Verification items for the finished model (mm, model axes). Give positions to 0.01 mm unless a question says otherwise; leave off trailing zeros. Loops run counter-clockwise (first coordinate to the right, second up) from the corner with the lowest first, then second, coordinate; pieces in that order, holes last. Notation, with made-up numbers: (82, 52) - (106, 52) arc R15 ccw to (106, 72) - close; hole circle Ø2 at (6, -16.75). An arc over 180 degrees is marked (long way). One line per item, written item: value. Start each with the question number.
1. Sectioned sample at D-D (x = 1.95). Count the separate pieces of the cut face and the enclosed holes in it, plus the area to 3 significant figures.
2. Scan lines: L1, parallel to Z at x = 2.25, y = 41; L2, parallel to Y at x = 0.5, z = -64 (3 decimals); L3, parallel to Z at x = 1.9, y = 6.5 (3 decimals). Record each from-to range of solid material in increasing order. Write a range as [from, to].
3. Sectioned sample at C-C (z = -80.5). Record the cut outline in (x, y).
4. Gauge pin test, flat ends, axial feed: pin 1 (1.5 mm diameter, centred on x = 2, y = 7, fed in from +Z); pin 2 (1.5 mm diameter, centred on x = 2, y = 7, fed in from -Z); pin 3 (0.9 mm diameter, centred on x = 1, y = 6, fed in from +Z). Record the tip position at first contact, or that the pin passes through.
5. Sectioned sample at B-B (y = 6.5). Record the cut outline in (x, z) (3 decimals), plus the area to 3 significant figures.
6. Sectioned sample at A-A (z = -11). Record the cut outline in (x, y), plus the area to 3 significant figures.
Autodesk Inventor part; units mm, degrees
ref_plane "YZ Plane" through (0, 0, 0) normal (1, 0, 0) x (0, 1, 0)
ref_plane "XZ Plane" through (0, 0, 0) normal (0, 1, 0) x (-1, 0, 0)
ref_plane "XY Plane" through (0, 0, 0) normal (0, 0, 1) x (1, 0, 0)
sketch "Sketch1" plane through (0, 0, 0) normal (1, 0, 0) x (0, 1, 0)
  line L0 (18.4717, 7.7423) -> (30.7168, -6.8509)
  line L1 (75.6155, -60.3591) -> (73.4706, -62.1589)
  line L2 (73.4706, -62.1589) -> (61.2255, -47.5657) construction
  line L3 (16.3268, 5.9425) -> (18.4717, 7.7423)
  line L4 (30.7168, -6.8509) -> (28.5719, -8.6507)
  line L5 (63.3704, -45.7659) -> (61.2255, -47.5657)
  line L6 (30.7168, -6.8509) -> (63.3704, -45.7659) construction
  line L7 (63.3704, -45.7659) -> (75.6155, -60.3591)
  line L8 (61.2255, -47.5657) -> (45.895, -29.2956)
  line L9 (28.5719, -8.6507) -> (16.3268, 5.9425) construction
  arc A0 (2.8222, 0.1573) -> (16.3268, 5.9425) centre (0, 25.4) ccw
  line L10 (0, -2.9981) -> (0, -85.6796)
  arc A1 (3.2657, -88.8533) -> (73.4706, -62.1589) centre (0, 25.4) ccw
  arc A2 (2.8222, 0.1573) -> (0, -2.9981) centre (3.175, -2.9981) ccw
  arc A3 (0, -85.6796) -> (3.2657, -88.8533) centre (3.175, -85.6796) ccw
  line L11 (5, -6.2388) -> (8, -6.2388)
  line L12 (8, -6.2388) -> (8, -25.2888)
  line L13 (8, -82.4388) -> (5, -82.4388)
  line L14 (5, -82.4388) -> (5, -63.3888)
  line L15 (8, -25.2888) -> (5, -25.2888)
  line L16 (8, -63.3888) -> (5, -63.3888)
  line L17 (8, -25.2888) -> (8, -63.3888) construction
  line L18 (5, -25.2888) -> (5, -6.2388)
  line L19 (5, -63.3888) -> (5, -25.2888) construction
  line L20 (8, -63.3888) -> (8, -82.4388)
  circle A4 centre (6.5, -44.3388) radius 1.5
  line L21 (51.7389, -22.3686) -> (29.8853, -40.706)
  line L22 (43.9024, -26.9208) -> (40.0722, -30.1348)
  line L23 (40.0722, -30.1348) -> (39.6966, -29.6872)
  line L24 (39.333, -29.2538) -> (38.8996, -29.6174) construction
  line L25 (37.4945, -30.7965) -> (38.2337, -31.6775)
  line L26 (38.2337, -31.6775) -> (36.7016, -32.963)
  line L27 (36.7016, -32.963) -> (37.6979, -34.1504)
  arc A5 (39.6966, -29.6872) -> (39.333, -29.2538) centre (39.2981, -29.6523) ccw
  line L28 (39.6966, -29.6872) -> (39.333, -29.2538) construction
  line L29 (38.8996, -29.6174) -> (37.4945, -30.7965)
  arc A6 (39.333, -29.2538) -> (38.8996, -29.6174) centre (39.2981, -29.6523) ccw
  line L30 (45.895, -29.2956) -> (42.0648, -32.5095)
  line L31 (42.0648, -32.5095) -> (42.4404, -32.9571)
  line L32 (40.9655, -34.9332) -> (40.2263, -34.0522)
  line L33 (40.2263, -34.0522) -> (38.6942, -35.3378)
  line L34 (38.6942, -35.3378) -> (37.6979, -34.1504)
  arc A7 (42.804, -33.3905) -> (42.4404, -32.9571) centre (42.4055, -33.3556) ccw
  line L35 (42.3707, -33.7541) -> (40.9655, -34.9332)
  arc A8 (42.3707, -33.7541) -> (42.804, -33.3905) centre (42.4055, -33.3556) ccw
  line L36 (43.9024, -26.9208) -> (28.5719, -8.6507)
  line L37 (45.895, -29.2956) -> (43.9024, -26.9208)
  line L38 (15.875, -26.9394) -> (15.875, -67.9256)
  line L39 (21.4822, -24.8986) -> (47.8276, -56.2958)
  arc A9 (19.685, -71.0364) -> (46.9085, -61.1279) centre (0, 25.4) ccw
  arc A10 (21.4822, -24.8986) -> (15.875, -26.9394) centre (19.05, -26.9394) ccw
  arc A11 (15.875, -67.9256) -> (19.685, -71.0364) centre (19.05, -67.9256) ccw
  arc A12 (46.9085, -61.1279) -> (47.8276, -56.2958) centre (45.3954, -58.3366) ccw
  point P0 (0, 0)
  point P1 (0, 0)
  point P2 (0, -88.9)
  point P3 (75.5935, -60.3328)
  point P4 (0, -44.3388)
  point P5 (5, -44.3388)
  point P6 (6.5, -25.2888)
  point P7 (44.8987, -28.1082)
  point P8 (15.875, -71.7363)
  point P9 (50.2771, -59.215)
  point P10 (15.875, -71.7363)
  dimension "d0" = 2.8
  dimension "d1" = 88.9
  dimension "d2" = 19.05
  dimension "d3" = 19.05
  dimension "d4" = 40
  dimension "d5" = 25.4
  dimension "d6" = 3.175
  dimension "d7" = 3
  dimension "d8" = 76.2
  dimension "d9" = 5
  dimension "d10" = 19.05
  dimension "d11" = 3
  dimension "d12" = 3.1
  dimension "d13" = 5.4
  dimension "d14" = 5
  dimension "d15" = 0.4
  dimension "d16" = 2.4
  dimension "d17" = 2
  dimension "d22" = 15.875
  dimension "d23" = 15.875
  dimension "d24" = 15.875
  dimension "d25" = 3.175
extrude "Extrusion1" add sketch "Sketch1" along normal blind 3 contours L0 L4 L36 L22 L23 A5 A6 L29 L25 L26 L27 L34 L33 L32 L35 A8 A7 L31 L30 L8 L5 L7 L1 A1 A3 L10 A2 A0 L3
equation "\"d3\" = d2"
equation "\"d23\" = d22"
equation "\"d24\" = d22"
properties part number "SideMount"
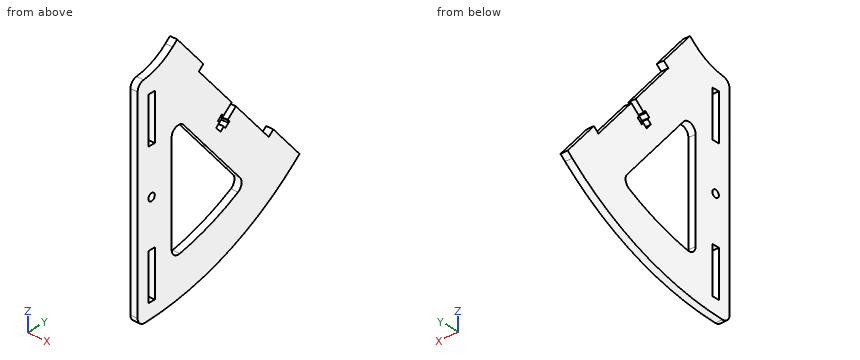
Results are:
1. separate pieces: 1
1. enclosed holes: 4
1. area: 3,340 mm^2
2. L1: z = [-81.29, -64.08], [-48.16, -34.9], [-29.36, -23.46]
2. L2: y = [0, 5], [8, 15.875], [41.172, 71.219]
2. L3: z = [-88.715, -82.439], [-63.389, -45.839], [-42.839, -25.289], [-6.239, 0.846]
3. outline: (0, 0) - (3, 0) - (3, 5) - (0, 5) - close; (0, 8) - (3, 8) - (3, 43.01) - (0, 43.01) - close
4. pin 1: stops at z = 1.21
4. pin 2: stops at z = -88.73
4. pin 3: stops at z = 0.83
5. outline: (0, -88.715) - (3, -88.715) - (3, -82.439) - (0, -82.439) - close; (0, -63.389) - (3, -63.389) - (3, -45.839) - (0, -45.839) - close; (0, -42.839) - (3, -42.839) - (3, -25.289) - (0, -25.289) - close; (0, -6.239) - (3, -6.239) - (3, 0.846) - (0, 0.846) - close
5. area: 145 mm^2
6. outline: (0, 0) - (3, 0) - (3, 5) - (0, 5) - close; (0, 8) - (3, 8) - (3, 30.54) - (0, 30.54) - close
6. area: 82.6 mm^2
